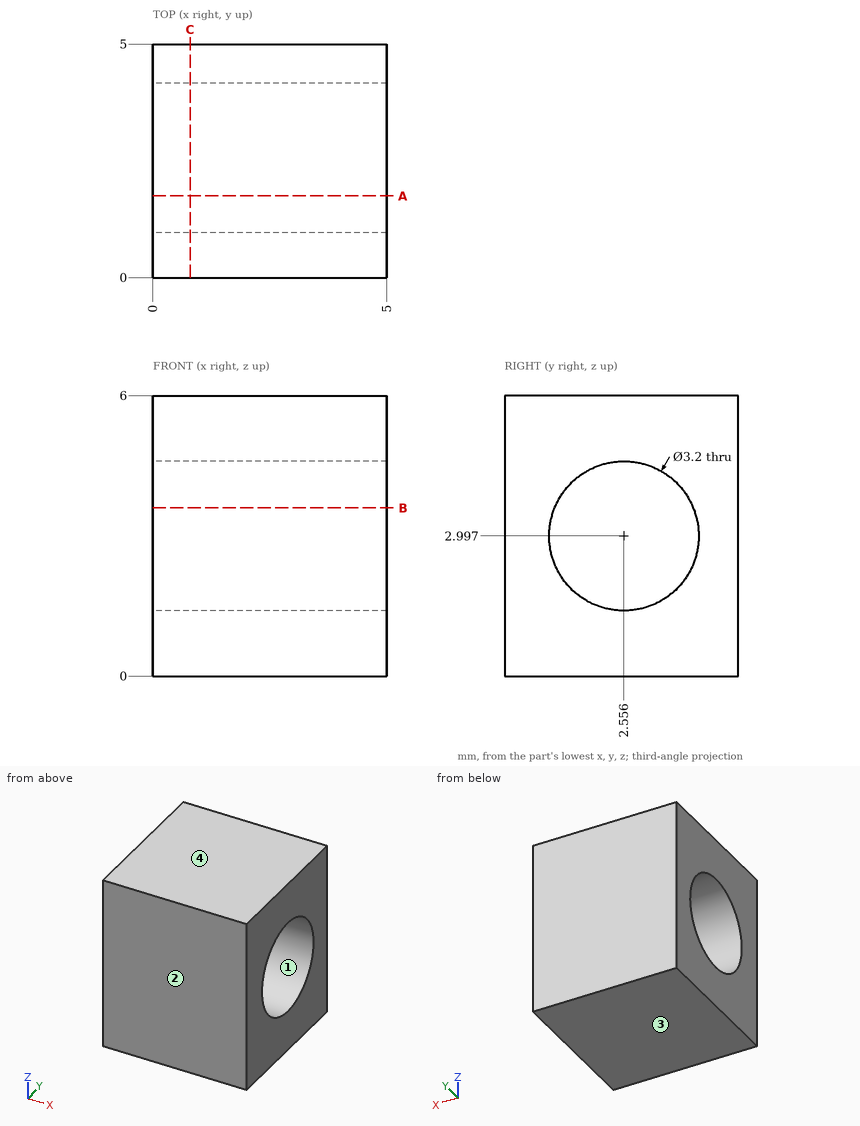
Verification items for this drawing (mm, ordinates from the low corner). Give positions to 0.01 mm unless a question says otherwise; leave off trailing zeros. Loops run counter-clockwise (first coordinate to the right, second up) from the corner with the lowest first, then second, coordinate; pieces in that order, holes last. Notation, with made-up numbers: M 53,60.5 L 64,60.5 A33 cw 64,98.5 Z; hole C 28,-39.5 d3. An arc over 180 degrees is marked long. Answer as a JSON object with one key per item and string values. Group by question number.
Q1. Cross-section at C-C on x = 0.8. Record the cut outline in (y, z).
Q2. Cross-section at A-A on y = 1.75. Record the cut outline in (x, z) (1 decimal).
Q3. Cross-section at B-B on z = 3.6. Record the cut outline in (x, y), then the cut area to 3 significant figures.
Q4. Release check for a two-part mould opening along Z. For the marked faces 1, 2, 3 and 4 record: released by +Z, released by -Z, zero draft, split by the parting line, or undercut.
Q5. Material ranges on line 1 along Z through (x, y) = (3.35, 2.5); line 2 along Y through (x, z) = (0.85, 4.05); line 3 along Y through (x, z) = (1.3, 4.3) (1 decimal), recorded low to high. Write a range as [from, to].
Evaluation:
{
 "1": {"outline": "M 0,0 L 5,0 L 5,6 L 0,6 Z; hole C 2.56,3 d3.2"},
 "2": {"outline": "M 0,0 L 5,0 L 5,1.6 L 0,1.6 Z; M 0,4.4 L 5,4.4 L 5,6 L 0,6 Z"},
 "3": {"outline": "M 0,0 L 5,0 L 5,1.07 L 0,1.07 Z; M 0,4.04 L 5,4.04 L 5,5 L 0,5 Z", "area": "10.2 mm2"},
 "4": {"face 1": "undercut", "face 2": "zero draft", "face 3": "released by -Z", "face 4": "released by +Z"},
 "5": {"line 1": "z = [0, 1.4], [4.6, 6]", "line 2": "y = [0, 1.35], [3.76, 5]", "line 3": "y = [0, 1.6], [3.5, 5]"}
}
